Here's the drawing with two shaded views (mm, measured from the low corner). I have some questions. A direction names the side the tool comes from. Round coordinates to 2 decimals unless told otherwise and drop trailing zeros. Loops run counter-clockwise (first coordinate to the right, second up) from the corner with the lowest first, then second, coordinate; pieces in that order, holes last.
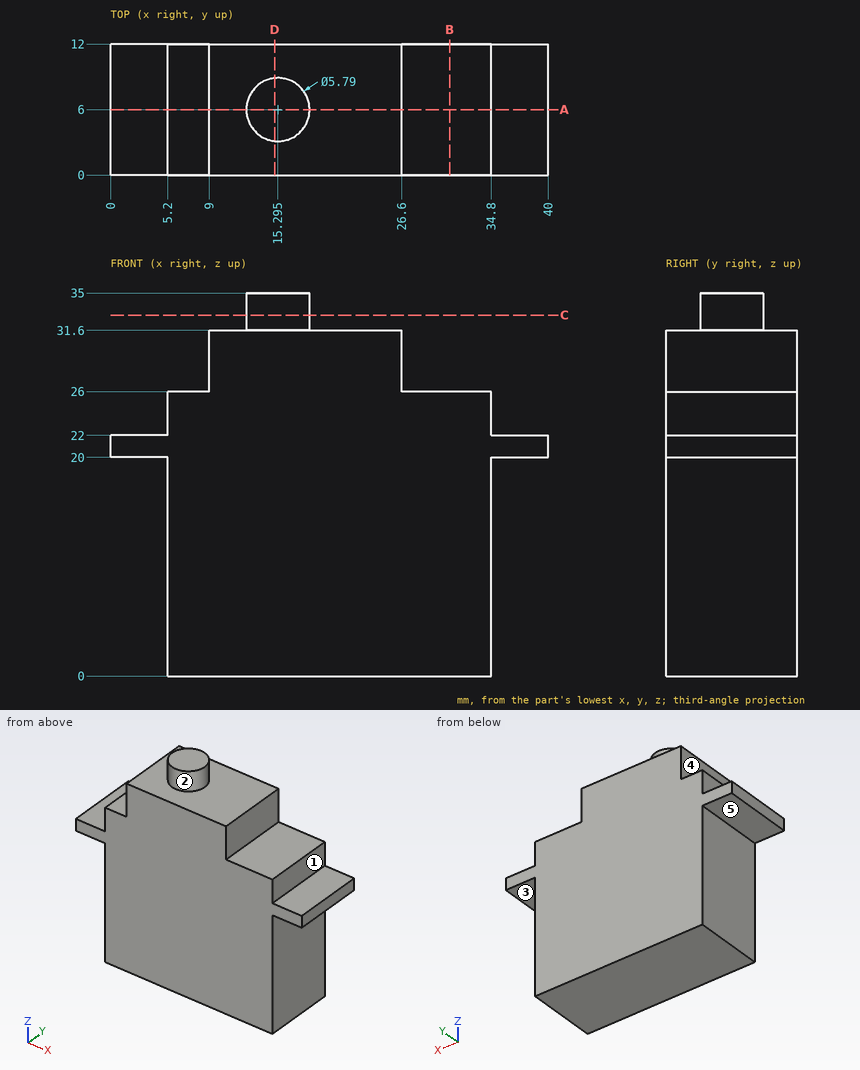
(1) For the marked faces 1, 2, 3, 4 and 5, which set-ups out of +Z, -Z, +X, -X, +Y, -Y let a thin tool reach every point of the face, with its end or its side?
Worked answers:
face 1: +Z, +X, +Y, -Y
face 2: +Z
face 3: -Z, +X, +Y, -Y
face 4: +Z, -X, +Y, -Y
face 5: -Z, -X, +Y, -Y
(2) If we section it at A-A, the plane y = 6: List the corners of the cut face in (x, z) for me, then the cut area to 3 significant figures.
Worked answers:
outline: (0, 20) - (5.2, 20) - (5.2, 0) - (34.8, 0) - (34.8, 20) - (40, 20) - (40, 22) - (34.8, 22) - (34.8, 26) - (26.6, 26) - (26.6, 31.6) - (18.19, 31.6) - (18.19, 35) - (12.4, 35) - (12.4, 31.6) - (9, 31.6) - (9, 26) - (5.2, 26) - (5.2, 22) - (0, 22) - close
area: 909 mm2
(3) If we section it at D-D, the plane x = 15: List the corners of the cut face in (y, z) for me.
Worked answers:
outline: (0, 0) - (12, 0) - (12, 31.6) - (8.88, 31.6) - (8.88, 35) - (3.12, 35) - (3.12, 31.6) - (0, 31.6) - close
(4) If we section it at B-B, the plane x = 31: List the corners of the cut face in (y, z) for me, then the cut area to 3 significant figures.
Worked answers:
outline: (0, 0) - (12, 0) - (12, 26) - (0, 26) - close
area: 312 mm2
(5) If we section it at C-C, the plane z = 33: List the corners of the cut face in (x, y) for me (3 decimals).
Worked answers:
outline: circle Ø5.79 at (15.295, 6)
(6) If I drill on line 1 (X direction, y = 8.5, z = 28.5); line 2 (Z direction, x = 34.5, y = 1.5); line 3 (X direction, y = 3.75, z = 11), over which ranges is the centre line in solid material (lowest first)?
Worked answers:
line 1: x = 9 to 26.6
line 2: z = 0 to 26
line 3: x = 5.2 to 34.8
(7) Will these pins go through, and if not, where does the flat tip stop? P1, Ø1.2, axis at y = 6.5, z = 24.5, coming from the +X side; P2, Ø3, axis at x = 6.5, y = 6, coming from the +Z side; P3, Ø4, axis at x = 37.5, y = 5, coming from the +Z side; P4, Ø10, axis at x = 4, z = 24, coming from the -Y side.
Worked answers:
P1: stops at x = 34.8
P2: stops at z = 26
P3: stops at z = 22
P4: stops at y = 0
